Here's how the part is built. I have some questions about the finished solid (model axes, mm). A direction names the side the tool comes from. Round coordinates to 2 decimals unless told otherwise and drop trailing zeros. Loops run counter-clockwise (first coordinate to the right, second up) from the corner with the lowest first, then second, coordinate; pieces in that order, holes last. Notation, with made-up numbers: M 56.25,9 L 79.25,9 A8 ccw 79.25,24 Z; hole C 82,72.25 d1. An arc over 180 degrees is marked long. Answer as a JSON object with one key per item and string values.
from build123d import *

# Parameters (mm, degrees)
SZKIC1_W                    = 10
SZKIC1_H                    = 20
DODANIE_WYCI_GNI_CIE1_DEPTH = 6


with BuildPart() as part:
    # Szkic1 → Dodanie-wyciągnięcie1 (new body)
    with BuildSketch(Plane.XY):
        with Locations((5, 10)):
            Rectangle(SZKIC1_W, SZKIC1_H)
        with BuildLine():
            Line((10, 20), (10, 14.482972118))
            Line((10, 14.482972118), (11.5, -2))
            Line((11.5, -2), (13.491769539, -1.818742986))
            ThreePointArc((13.491769539, -1.818742986), (15.302282063, 0.354283567), (13.129255511, 2.164796091))
            Line((13.129255511, 2.164796091), (11.635428357, 2.028853331))
            Line((11.635428357, 2.028853331), (10, 20))
        make_face()
    extrude(amount=DODANIE_WYCI_GNI_CIE1_DEPTH)


solid = part.part
Item 1: If I drill on L1, parallel to Y at x = 8, z = 2.55; L2, parallel to X at y = 8.25, z = 0.5; L3, parallel to Y at x = 13.5, z = 4.75, over which ranges is the centre line in solid material (lowest first)? Write a range as from..to.
Solution:
{"L1": "y = 0..20", "L2": "x = 0..10, 10.57..11.07", "L3": "y = -1.82..2.16"}
Item 2: We'd pull the mould along X, two halves only. Please class faces 1 (the face through (6, 9, 0)), 2 (the face through (0, 10, 3)), 3 (the face through (10.74, 6.36, 2.96)): +X half, -X half, draft (parallel to the pull), parting line (faces both ways), or undercut.
Solution:
{"face 1": "draft", "face 2": "-X half", "face 3": "undercut"}
Item 3: For faces 4 (the face through (5, 0, 3)), 5 (the face through (12.48, -1.91, 2.96)), 6 (the face through (12.4, 2.1, 3)), which set-ups out of +Z, -Z, +X, -X, +Y, -Y let a thin tool reach every point of the face, with its end or its side?
Solution:
{"face 4": "+Z, -Z, -X, -Y", "face 5": "+Z, -Z, +X, -Y", "face 6": "+Z, -Z, +Y"}
Item 4: I want a section at D-D on y = 6.25. List the corners of the cut face in (x, z) for me, plus the area to 3 significant figures.
Solution:
{"outline": "M 0,0 L 10,0 L 10,6 L 0,6 Z; M 10.75,0 L 11.25,0 L 11.25,6 L 10.75,6 Z", "area": "63.0 mm2"}
Item 5: I want a section at C-C on x = 6.75. List the corners of the cut face in (y, z) for me.
Solution:
{"outline": "M 0,0 L 20,0 L 20,6 L 0,6 Z"}
Item 6: I want a section at B-B on y = 0.25. List the corners of the cut face in (x, z) for me.
Solution:
{"outline": "M 0,0 L 10,0 L 10,6 L 0,6 Z; M 11.3,0 L 15.31,0 L 15.31,6 L 11.3,6 Z"}
Item 7: For P1, Ø1, axis at y = 11.5, z = 1.5, coming from the +X side; P2, Ø3, axis at x = 3, z = 5.5, coming from the -Y side; P3, Ø3, axis at y = 7, z = 3.5, coming from the +X side, each with a flat end and sliding along its axis, tell me the tip position at first contact or that it passes through.
Solution:
{"P1": "stops at x = 10.82", "P2": "stops at y = 0", "P3": "stops at x = 11.32"}
Item 8: I want a section at A-A on z = 2.75. List the corners of the cut face in (x, y) for me.
Solution:
{"outline": "M 0,0 L 10,0 L 10,14.48 L 11.5,-2 L 13.49,-1.82 A2 ccw 13.13,2.16 L 11.64,2.03 L 10,20 L 0,20 Z"}
